The listing builds one solid part. Answer for the finished solid, in the listing's coordinates (mm). Face numbers are marked on the shaded views. Coordinates: 2 decimals unless noted, no trailing zeros. Write each loop counter-clockwise with the first axis right and the second up, starting at its lowest first coordinate (ties: lowest second). Pieces come first, ordered by that corner, then holes.
(1) The part is cut by section B-B on y = 4. Determine the outline of the cut face in (x, z), plus the area to 3 significant figures.
(2) Given P1, Ø4, axis at y = 14.5, z = 40, coming from the +X side; P2, Ø7, axis at x = 0, z = 0, coming from the +Y side; P3, Ø10, axis at x = 34.5, z = 33, coming from the -Y side; P4, Ø12, axis at x = -3, z = 0, coming from the -Y side, each flat-ended and moving along its own axis, determine where each tip first touches the part or whether it passes through.
(3) The part is cut by section C-C on z = 0. Give the number of separate pieces and of enclosed holes in the cut face, plus the area to 3 significant figures.
(4) Straight lines are drawn through the part: line 1 (Y direction, x = -58.5, z = 0); line 2 (Z direction, x = -10, y = 18); line 3 (X direction, y = 2, z = 21.5). For each, find the intervals that lie inside material, in ascending order.
(5) For a pull along Z with two mould halves and no side action, classify the marked faces 1, 2, 3 and 4 as +Z half, -Z half, draft (parallel to the pull), parting line (faces both ways), or undercut.
(6) The part is cut by section A-A on y = 20. Determine the outline of the cut face in (x, z), plus the area to 3 significant figures.
from build123d import *

# Parameters (mm, degrees)
SKETCH2_R               = 3.35
CUT_EXTRUDE1_DEPTH      = 25
CIRPATTERN1_COUNT       = 4
SKETCH5_R               = 53.5
SKETCH5_R_2             = 29
CUT_EXTRUDE4_DEPTH      = 28
CUT_EXTRUDE5_REACH      = 145.217
CUT_EXTRUDE5_END_RADIUS = 53.5
SKETCH6_R               = 2.1
CIRPATTERN2_COUNT       = 6
CHAMFER1_SIZE           = 2
FILLET2_R               = 1
FILLET3_R               = 5


with BuildPart() as part:
    # Sketch1 → Revolve1 (revolve)
    with BuildSketch(Plane(origin=(0, 0, 0), x_dir=(0, 0, -1), z_dir=(1, 0, 0)), mode=Mode.PRIVATE) as revolve1_sk:
        Polygon((-24, 0), (-61.5, 0), (-61.5, 40), (-6, 40), (-6, 35), (-13, 35), (-13, 7.5), (-24, 7.5), align=None)
    revolve(revolve1_sk.sketch.rotate(Axis((0, 0, 0), (0, 1, 0)), 180), axis=Axis((0, 0, 0), (0, 1, 0)))

    # Sketch2 → Cut-Extrude1 (cut)
    with BuildSketch(Plane(origin=(0, 40, 0), x_dir=(1, 0, 0), z_dir=(0, 1, 0))):
        with Locations(Location((-32.5, 32.5, 0), (0, 0, 270))):
            Circle(SKETCH2_R)
    cut_extrude1 = extrude(amount=-CUT_EXTRUDE1_DEPTH, mode=Mode.SUBTRACT)

    # CirPattern1: Cut-Extrude1 ×4 about axis
    cirpattern1_axis = Axis((0, 0, 0), (0, 1, 0))
    for i in range(1, CIRPATTERN1_COUNT):
        add(cut_extrude1.rotate(cirpattern1_axis, i * 360 / CIRPATTERN1_COUNT), mode=Mode.SUBTRACT)

    # Sketch5 → Cut-Extrude4 (cut)
    with BuildSketch(Plane.XZ):
        with Locations(Location((0, 0, 0), (0, 0, 270))):
            Circle(SKETCH5_R)
        with Locations(Location((0, 0, 0), (0, 0, 270))):
            Circle(SKETCH5_R_2, mode=Mode.SUBTRACT)
    extrude(amount=-CUT_EXTRUDE4_DEPTH, mode=Mode.SUBTRACT)

    # Cut-Extrude5: up to this cylinder (the profile starts outside it)
    cut_extrude5_end = Plane(origin=(0, 20, 0), z_dir=(0, -1, 0)) * Cylinder(CUT_EXTRUDE5_END_RADIUS, 398.434, mode=Mode.PRIVATE)
    # Sketch6 → Cut-Extrude5 (cut, up to the surface)
    with BuildSketch(Plane(origin=(61.5, 0, 0), x_dir=(0, 0, -1), z_dir=(1, 0, 0)), mode=Mode.PRIVATE) as cut_extrude5_sk1:
        with Locations((0, 20)):
            Circle(SKETCH6_R)
    cut_extrude5_tool1 = extrude(cut_extrude5_sk1.sketch, amount=-CUT_EXTRUDE5_REACH, mode=Mode.PRIVATE) - cut_extrude5_end
    cut_extrude5 = cut_extrude5_tool1.solids().sort_by_distance((61.5, 20, 0))[0]
    add(cut_extrude5, mode=Mode.SUBTRACT)

    # CirPattern2: Cut-Extrude5 ×6 about axis
    cirpattern2_axis = Axis((0, 40, 0), (0, -1, 0))
    for i in range(1, CIRPATTERN2_COUNT):
        add(cut_extrude5.rotate(cirpattern2_axis, i * 360 / CIRPATTERN2_COUNT), mode=Mode.SUBTRACT)

    # Chamfer1
    chamfer1_edges = [part.edges().sort_by_distance(p)[0] for p in [
        (0, 0, 24),
        (0, 0, 53.5),
        (0, 0, 29),
        (0, 7.5, 13),
        (0, 35, 6),
        (0, 40, 6),
        (0, 40, 61.5),
        (0, 0, 61.5),
    ]]
    chamfer(chamfer1_edges, length=CHAMFER1_SIZE)

    # Fillet2
    fillet2_edges = [part.edges().sort_by_distance(p)[0] for p in [
        (0, 28, 53.5),
        (0, 7.5, 24),
        (0, 35, 13),
    ]]
    fillet(fillet2_edges, radius=FILLET2_R)

    # Fillet3
    fillet3_edges = [part.edges().sort_by_distance(p)[0] for p in [
        (0, 28, 29),
    ]]
    fillet(fillet3_edges, radius=FILLET3_R)


solid = part.part
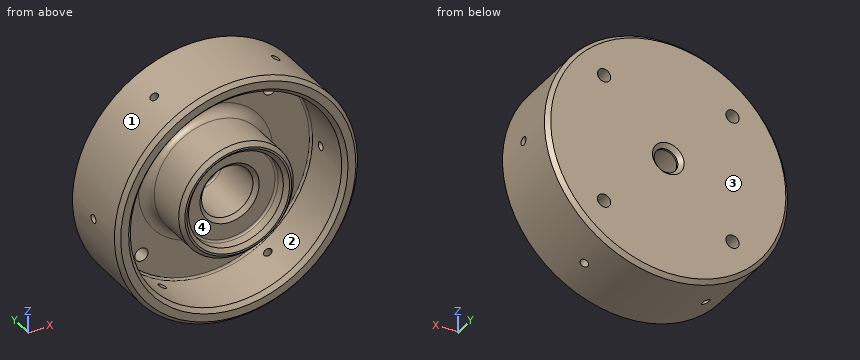
Model answer:
1. outline: circle Ø123 at (0, 0); circle Ø58 at (0, 0); hole circle Ø107 at (0, 0); hole circle Ø48 at (0, 0)
1. area: 3,720 mm2
2. P1: stops at x = 48.36
2. P2: passes through
2. P3: stops at y = 27.97
2. P4: stops at y = 35
3. separate pieces: 4
3. enclosed holes: 0
3. area: 2,330 mm2
4. line 1: y = 0 to 17.9, 22.1 to 40
4. line 2: z = -60.68 to -52.56, -27.22 to -8.31, 8.31 to 27.22, 52.56 to 60.68
4. line 3: x = -57.62 to -48.99, -19.46 to -10.67, 10.67 to 19.46, 48.99 to 57.62
5. face 1: parting line
5. face 2: undercut
5. face 3: draft
5. face 4: undercut
6. outline: (-61.46, -2.1) arc R61.5 ccw to (-32.55, -52.18) - (-28.55, -45.25) arc R53.5 cw to (-53.46, -2.1) - close; (-61.46, 2.1) - (-53.46, 2.1) arc R53.5 cw to (-28.55, 45.25) - (-32.55, 52.18) arc R61.5 ccw to start; circle Ø58 at (0, 0); (-28.91, -54.28) arc R61.5 ccw to (28.91, -54.28) - (24.91, -47.35) arc R53.5 cw to (-24.91, -47.35) - close; (-28.91, 54.28) - (-24.91, 47.35) arc R53.5 cw to (24.91, 47.35) - (28.91, 54.28) arc R61.5 ccw to start; (28.55, -45.25) - (32.55, -52.18) arc R61.5 ccw to (61.46, -2.1) - (53.46, -2.1) arc R53.5 cw to start; (28.55, 45.25) arc R53.5 cw to (53.46, 2.1) - (61.46, 2.1) arc R61.5 ccw to (32.55, 52.18) - close; hole circle Ø26 at (0, 0)
6. area: 4,800 mm2
